Check sheet for the modelled part. Datum: model origin and axes. Units: mm. Face numbers are marked on the shaded views. A direction names the side the tool comes from. Coordinates: 2 decimals unless noted, no trailing zeros. Loops run counter-clockwise (first coordinate to the right, second up) from the corner with the lowest first, then second, coordinate; pieces in that order, holes last. Notation, with made-up numbers: M -4.75,-31.75 L 0.25,-31.75 A31 cw 0.25,-1.75 Z; hole C 46,24.5 d10. An arc over 180 degrees is marked long. Answer as CSV lines item,"result". Start each with the question number.
Autodesk Inventor part; units mm, degrees
ref_plane "YZ Plane" through (0, 0, 0) normal (1, 0, 0) x (0, 1, 0)
ref_plane "XZ Plane" through (0, 0, 0) normal (0, 1, 0) x (-1, 0, 0)
ref_plane "XY Plane" through (0, 0, 0) normal (0, 0, 1) x (1, 0, 0)
sketch "スケッチ1" plane through (0, 0, 0) normal (0, 0, 1) x (1, 0, 0)
  circle A0 centre (0, 0) radius 2.5
  dimension "d0" = 5
extrude "押し出し1" add sketch "スケッチ1" along normal blind 6
sketch "スケッチ2" plane through (0, 0, 6) normal (0, 0, 1) x (1, 0, 0)
  circle A0 centre (0, 0) radius 2.5
  circle A1 centre (0, 0) radius 5
  dimension "d3" = 10
extrude "押し出し2" add sketch "スケッチ2" along normal blind 3.4 contours A0 | A1
fillet "フィレット1" radius 3.4 1 edges at (-5, 0, 9.4)
thread "ねじ1"
sketch "スケッチ3" plane through (0, 0, 0) normal (0, 0, -1) x (-1, 0, 0)
  circle A0 centre (0, 0) radius 2.5
extrude "押し出し3" add sketch "スケッチ3" along normal blind 10
properties part number "SB　M5 16mmなべネジ" material "Steel, Mild"
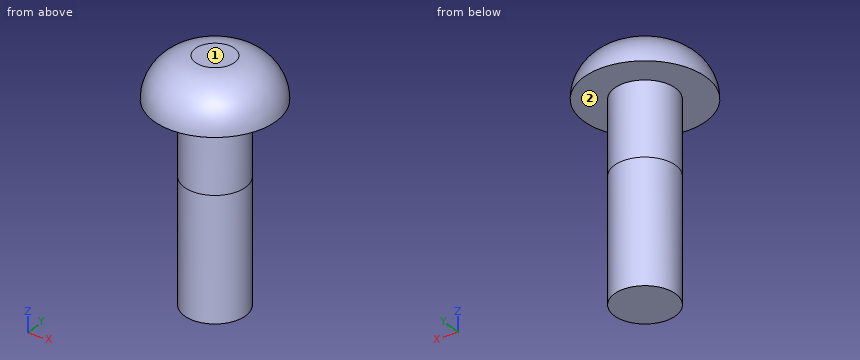
Item 1: Sectioned sample at A-A, the plane z = -5.75. Record the boundary of the cut face in (x, y).
Item 2: Go/stop test with flat-tipped pins: pin 1 (5 mm diameter, centred on x = -1.5, y = -2.5, fed in from -Z); pin 2 (4 mm diameter, centred on x = 3.5, y = 2, fed in from +Z); pin 3 (5 mm diameter, centred on y = 2, z = 2, fed in from -X); pin 4 (1 mm diameter, centred on x = -2.5, y = 3, fed in from -Z). Record where each tip stops, or that it passes through.
Item 3: Set-up check for the marked faces 1 and 2: record each of +Z, -Z, +X, -X, +Y, -Y from which the full face is reachable in a straight line by a thin tool's end or side.
Item 4: Material ranges on line 1 (X direction, y = -0.5, z = -4.75); line 2 (Y direction, x = -0.25, z = -5), recorded low to high. Write a range as from..to.
Reply:
1,outline,"C 0,0 d5"
2,pin 1,"z = -10"
2,pin 2,"z = 9.37"
2,pin 3,"x = -2.5"
2,pin 4,"z = 6"
3,face 1,"+Z, +X, -X, +Y, -Y"
3,face 2,"-Z"
4,line 1,"-2.45..2.45"
4,line 2,"-2.49..2.49"
